from build123d import *

# Parameters (mm, degrees)
SKETCH1_W                                         = 107.95
SKETCH1_H                                         = 12.7
BOSS_EXTRUDE1_DEPTH                               = 31.75
FILLET1_R                                         = 12.7
CSK_FOR_8_FLAT_HEAD_MACHINE_SCREW_100_D           = 4.4958
CSK_FOR_8_FLAT_HEAD_MACHINE_SCREW_100_DEPTH       = 19.05
CSK_FOR_8_FLAT_HEAD_MACHINE_SCREW_100_CSINK_D     = 8.4328
CSK_FOR_8_FLAT_HEAD_MACHINE_SCREW_100_CSINK_ANGLE = 100
CSK_FOR_8_FLAT_HEAD_MACHINE_SCREW_100_TIP         = 1.350674586
FILLET2_R                                         = 1.5875


with BuildPart() as part:
    # Sketch1 → Boss-Extrude1 (new, symmetric)
    with BuildSketch(Plane.XY):
        Rectangle(SKETCH1_W, SKETCH1_H)
    extrude(amount=BOSS_EXTRUDE1_DEPTH, both=True)

    # Fillet1
    fillet1_edges = [part.edges().sort_by_distance(p)[0] for p in [
        (-53.975, 0, 31.75),
        (53.975, 0, 31.75),
    ]]
    fillet(fillet1_edges, radius=FILLET1_R)

    # CSK for #8 Flat Head Machine Screw (100)1
    with Locations(Plane(origin=(0, 6.35, 0), x_dir=(1, 0, 0), z_dir=(0, 1, 0))):
        with Locations((-38.1, 25.4), (38.1, 25.4), (0, 25.4)):
            CounterSinkHole(CSK_FOR_8_FLAT_HEAD_MACHINE_SCREW_100_D / 2, CSK_FOR_8_FLAT_HEAD_MACHINE_SCREW_100_CSINK_D / 2, depth=CSK_FOR_8_FLAT_HEAD_MACHINE_SCREW_100_DEPTH, counter_sink_angle=CSK_FOR_8_FLAT_HEAD_MACHINE_SCREW_100_CSINK_ANGLE)
            with Locations((0, 0, -(CSK_FOR_8_FLAT_HEAD_MACHINE_SCREW_100_DEPTH + CSK_FOR_8_FLAT_HEAD_MACHINE_SCREW_100_TIP / 2))):  # 118° drill point
                Cone(0, CSK_FOR_8_FLAT_HEAD_MACHINE_SCREW_100_D / 2, CSK_FOR_8_FLAT_HEAD_MACHINE_SCREW_100_TIP, mode=Mode.SUBTRACT)

    # Fillet2
    fillet2_edges = [part.edges().sort_by_distance(p)[0] for p in [
        (0, 6.35, 31.75),
        (-53.975, 6.35, -6.35),
        (53.975, 6.35, -6.35),
        (50.255256121, 6.35, 28.030256121),
        (-50.255256121, 6.35, 28.030256121),
        (-53.975, 0, -31.75),
        (0, 6.35, -31.75),
        (53.975, 0, -31.75),
    ]]
    fillet(fillet2_edges, radius=FILLET2_R)


solid = part.part
CAD build for the part. Positions are in the model's coordinates, mm. Give positions to 0.01 mm unless a question says otherwise; leave off trailing zeros. Return JSON: item names as keys, results as strings.
Item 1: Drill centre lines: probe 1 along X at (y, z) = (-3.5, -25.4) (3 decimals); probe 2 along Z at (x, y) = (38.1, -2.25); probe 3 along X at (y, z) = (-4, -26.5) (3 decimals). Where is each one in solid material? Low to high.
Answer below:
{"probe 1": "x = -53.975 to -40.348, -35.852 to -2.248, 2.248 to 35.852, 40.348 to 53.975", "probe 2": "z = -31.75 to -27.65, -23.15 to 31.75", "probe 3": "x = -53.975 to -40.06, -36.14 to -1.96, 1.96 to 36.14, 40.06 to 53.975"}
Item 2: Band-saw the part on A-A (y = 0.25). Give the number of separate pieces and of enclosed holes in the cut face, then the cut area to 3 significant figures.
Answer below:
{"separate pieces": "1", "enclosed holes": "3", "area": "6,740 mm2"}
Item 3: Two-plate mould, pull along X, no slides. Class faces 1 (the flat face through (-1, -1, -31.75)), 2 (the cylindrical face through (0.487, -0.903, -23.206)), 3 (the flat face through (-53.975, -1, -5)): +X half, -X half, draft (parallel to the pull), parting line (faces both ways), or undercut.
Answer below:
{"face 1": "draft", "face 2": "undercut", "face 3": "-X half"}
